Work out the finished part from the listing and answer in its coordinate system (mm). Round coordinates to 2 decimals unless told otherwise and drop trailing zeros. Loops run counter-clockwise (first coordinate to the right, second up) from the corner with the lowest first, then second, coordinate; pieces in that order, holes last.
from build123d import *

# Parameters (mm, degrees)
PAD_DEPTH     = 4.763
SKETCH001_R   = 2
SKETCH001_R_2 = 3
POCKET_DEPTH  = 4.764
FILLET_R      = 5


with BuildPart() as part:
    # Sketch → Pad (new body)
    with BuildSketch(Plane.XY):
        with BuildLine():
            ThreePointArc((75.749521, 0), (0, 14.9), (-75.749521, 0))
            Line((-104.25, 0), (-75.749521, 0))
            Line((-104.25, 0), (-104.25, 30.01692))
            ThreePointArc((104.25, 30.01692), (0, 55), (-104.25, 30.01692))
            Line((104.25, 30.01692), (104.25, 0))
            Line((75.749521, 0), (104.25, 0))
        make_face()
    extrude(amount=PAD_DEPTH)

    # Sketch001 → Pocket (cut, through all)
    with BuildSketch(Plane.XY.offset(4.763)):
        with Locations((-31, 45.5)):
            Circle(SKETCH001_R)
        with Locations((36, 45.5)):
            Circle(SKETCH001_R)
        with Locations((36, 18)):
            Circle(SKETCH001_R)
        with Locations((-31, 18)):
            Circle(SKETCH001_R)
        with Locations((-90, 14.25)):
            Circle(SKETCH001_R_2)
        with Locations((-86, 32.75)):
            Circle(SKETCH001_R_2)
        with Locations((86, 32.75)):
            Circle(SKETCH001_R_2)
        with Locations((90, 14.25)):
            Circle(SKETCH001_R_2)
    extrude(amount=-POCKET_DEPTH, mode=Mode.SUBTRACT)

    # Fillet
    fillet_edges = [part.edges().sort_by_distance(p)[0] for p in [
        (-104.25, 30.01692, 2.3815),
        (-104.25, 0, 2.3815),
        (104.25, 30.01692, 2.3815),
        (-75.749521, 0, 2.3815),
        (75.749521, 0, 2.3815),
        (104.25, 0, 2.3815),
    ]]
    fillet(fillet_edges, radius=FILLET_R)


solid = part.part
Item 1: Section B-B, the plane x = 36 is taken. Give the vertices of the cut face in (y, z), plus the area to 3 significant figures.
Item 2: Determine the mould class of faces 1 (the face through (-29.092, 18.601, 2.415)), 2 (the face through (1, 28, 4.763)), 3 (the face through (102.75, 1.43, 2.41)) for opening direction X: pulls with the +X half, pulls with the -X half, needs draft (parallel to the pull), parting line crosses it, or undercut.
Item 3: Section C-C, the plane x = -31 is taken. Give the vertices of the cut face in (y, z), plus the area to 3 significant figures.
Item 4: Section A-A, the plane z = 2.55 is taken. State how many separate pieces and enclosed holes the cut face has, plus the area to 3 significant figures.
Item 5: Straight lines are drawn through the part: line 1 (X direction, y = 15, z = 3.55); line 2 (Y direction, x = 36, z = 3.45); line 3 (X direction, y = 31, z = 3.5). For each, find the intervals that lie inside material, in ascending order.
Item 6: Each of these flat-tipped pins is pushed along its axis until it touches: P1, Ø1.5, axis at y = 29.5, z = 3, coming from the -X side; P2, Ø3.5, axis at x = -31, y = 45.5, coming from the -Z side. Where does it stop, or does it pass through?
Answer below:
1. outline: (11.63, 0) - (16, 0) - (16, 4.76) - (11.63, 4.76) - close; (20, 0) - (43.5, 0) - (43.5, 4.76) - (20, 4.76) - close; (47.5, 0) - (52.17, 0) - (52.17, 4.76) - (47.5, 4.76) - close
1. area: 155 mm2
2. face 1: undercut
2. face 2: needs draft
2. face 3: pulls with the +X half
3. outline: (12.48, 0) - (16, 0) - (16, 4.76) - (12.48, 4.76) - close; (20, 0) - (43.5, 0) - (43.5, 4.76) - (20, 4.76) - close; (47.5, 0) - (52.9, 0) - (52.9, 4.76) - (47.5, 4.76) - close
3. area: 154 mm2
4. separate pieces: 1
4. enclosed holes: 8
4. area: 8,080 mm2
5. line 1: x = -104.25 to -92.9, -87.1 to 87.1, 92.9 to 104.25
5. line 2: y = 11.63 to 16, 20 to 43.5, 47.5 to 52.17
5. line 3: x = -102.15 to -88.44, -83.56 to 83.56, 88.44 to 102.15
6. P1: stops at x = -103.91
6. P2: passes through
